The model under review builds one solid part; all positions refer to its coordinate system, in mm. A direction names the side the tool comes from. Give positions to 0.01 mm unless a question says otherwise; leave off trailing zeros. Order: outer loops, then holes, each group sorted by start corner. A loop starts at its lowest first (then second) coordinate and runs counter-clockwise, first axis right, second up. Notation, with made-up numbers: (52.25, -37) - (93.25, -37) arc R16 ccw to (93.25, -6) - close; hole circle Ø10 at (59.25, 70.5). An arc over 180 degrees is marked (long way). Put each result on its own line as item: value.
```python
from build123d import *

# Parameters (mm, degrees)
SKETCH_1_R               = 9.5
EXTRUDE_1_DEPTH          = 108
SKETCH_2_R               = 6.35
EXTRUDE_2_DEPTH          = 11.5
SKETCH_3_R               = 11
EXTRUDE_3_DEPTH          = 8
SKETCH_4_R               = 9.5
EXTRUDE_4_DEPTH          = 1.6
SKETCH_5_R               = 11
EXTRUDE_5_DEPTH          = 14
SKETCH_6_R               = 9.5
EXTRUDE_6_DEPTH          = 4
SKETCH_7_R               = 14.25
EXTRUDE_7_DEPTH          = 16
CHAMFER_1_SIZE           = 1.5
CUT_EXTRUDE_1_DEPTH      = 195.148744523
CUT_EXTRUDE_1_DEPTH_BACK = 195.148744523
EXTRUDE_8_DEPTH          = 14
EXTRUDE_8_DEPTH_BACK     = 14
SKETCH_12_R              = 8
EXTRUDE_9_DEPTH          = 3.2
SKETCH_13_R              = 9.5
EXTRUDE_10_DEPTH         = 6.4
CHAMFER_2_SIZE           = 1.5
CHAMFER_2_SIZE2          = 2.598076211


with BuildPart() as part:
    # Sketch 1 → Extrude 1 (new body)
    with BuildSketch(Plane.XY):
        Circle(SKETCH_1_R)
    extrude(amount=EXTRUDE_1_DEPTH)

    # Sketch 2 → Extrude 2 (add)
    with BuildSketch(Plane.XY.offset(108)):
        Circle(SKETCH_2_R)
    extrude(amount=EXTRUDE_2_DEPTH)

    # Sketch 3 → Extrude 3 (add)
    with BuildSketch(Plane.XY.offset(119.5)):
        Circle(SKETCH_3_R)
    extrude(amount=EXTRUDE_3_DEPTH)

    # Sketch 4 → Extrude 4 (add)
    with BuildSketch(Plane.XY.offset(127.5)):
        Circle(SKETCH_4_R)
    extrude(amount=EXTRUDE_4_DEPTH)

    # Sketch 5 → Extrude 5 (add)
    with BuildSketch(Plane.XY.offset(129.1)):
        Circle(SKETCH_5_R)
    extrude(amount=EXTRUDE_5_DEPTH)

    # Sketch 6 → Extrude 6 (add)
    with BuildSketch(Plane.XY.offset(143.1)):
        Circle(SKETCH_6_R)
    extrude(amount=EXTRUDE_6_DEPTH)

    # Sketch 7 → Extrude 7 (add)
    with BuildSketch(Plane.XY.offset(147.1)):
        Circle(SKETCH_7_R)
    extrude(amount=EXTRUDE_7_DEPTH)

    # Chamfer 1
    chamfer_1_edges = [part.edges().sort_by_distance(p)[0] for p in [
        (-14.25, 0, 163.1),
    ]]
    chamfer(chamfer_1_edges, length=CHAMFER_1_SIZE)

    # Sketch 8 → Revolve 1 (revolve)
    with BuildSketch(Plane(origin=(0, 0, 0), x_dir=(0, 0, -1), z_dir=(1, 0, 0)), mode=Mode.PRIVATE) as revolve_1_sk:
        Polygon((-163.1, 6.35), (-164.7, 6.35), (-164.7, 9.5), (-166.3, 9.5), (-166.3, 6.35), (-167.9, 6.35), (-167.9, 9.5), (-169.5, 9.5), (-169.5, 6.35), (-171.1, 6.35), (-171.1, 9.5), (-172.7, 9.5), (-172.7, 6.35), (-193.1, 6.35), (-193.1, 0), (-163.1, 0), align=None)
    revolve(revolve_1_sk.sketch.rotate(Axis((0, 0, 193.1), (0, 0, -1)), 90), axis=Axis((0, 0, 193.1), (0, 0, -1)))

    # Sketch 9 → Cut-Extrude 1 (cut, two sides: drawn at the far end of the back side and taken through both)
    with BuildSketch(Plane(origin=(0, 0, 0), x_dir=(0, 0, -1), z_dir=(1, 0, 0)).offset(-CUT_EXTRUDE_1_DEPTH_BACK)):
        Polygon((-179.653682132, -6.35), (-188.546317868, 6.35), (-193.1, 6.35), (-193.1, -6.35), align=None)
    extrude(amount=CUT_EXTRUDE_1_DEPTH + CUT_EXTRUDE_1_DEPTH_BACK, mode=Mode.SUBTRACT)

    # Sketch 10 → Extrude 8 (add, two sides: drawn at the far end of the back side and taken through both)
    with BuildSketch(Plane(origin=(0, 0, 0), x_dir=(0, 0, -1), z_dir=(1, 0, 0)).offset(-EXTRUDE_8_DEPTH_BACK)):
        Polygon((-176.815579258, -10.403230962), (-191.384420742, 10.403230962), (-215.688134824, -6.614412844), (-201.119293341, -27.420874769), align=None)
    extrude(amount=EXTRUDE_8_DEPTH + EXTRUDE_8_DEPTH_BACK)

    # Sketch 12 → Extrude 9 (add)
    with BuildSketch(Plane(origin=(0, 76.095474781, 53.282625065), x_dir=(1, 0, 0), z_dir=(0, -0.8191520442889946, -0.5735764363510424))):
        with Locations(Location((0, 165.640569636, 0), (0, 0, 270))):
            Circle(SKETCH_12_R)
    extrude(amount=EXTRUDE_9_DEPTH)

    # Sketch 13 → Extrude 10 (add)
    with BuildSketch(Plane(origin=(0, 73.474188239, 51.447180469), x_dir=(1, 0, 0), z_dir=(0, -0.8191520442889944, -0.5735764363510425))):
        with Locations(Location((0, 165.640569636, 0), (0, 0, 270))):
            Circle(SKETCH_13_R)
    extrude(amount=EXTRUDE_10_DEPTH)

    # Chamfer 2
    chamfer_2_edges = [part.edges().sort_by_distance(p)[0] for p in [
        (-14.25, 0, 147.1),
    ]]
    chamfer_2_side = [part.faces().sort_by_distance(p)[0] for p in [
        (-13.846949135, 0, 147.1),
    ]]
    chamfer(chamfer_2_edges, length=CHAMFER_2_SIZE, length2=CHAMFER_2_SIZE2, reference=chamfer_2_side[0])


solid = part.part
```
(1) Take a section at B-B, the plane z = 157. Write out the cut boundary in (x, y), then the cut area to 3 significant figures.
The answers:
outline: circle Ø28.5 at (0, 0)
area: 638 mm^2
(2) Wall thickness on L1, parallel to Z at x = -6, y = -6; L2, parallel to Z at x = -5, y = 9; L3, parallel to Y at x = 5, z = 177: over which ranges is each line inside the solid? List them lowest first.
The answers:
L1: 0 to 108, 119.5 to 163.1, 164.7 to 166.3, 167.9 to 169.5, 171.1 to 172.7, 179.9 to 214.81
L2: 119.5 to 127.5, 129.1 to 143.1, 147.1 to 163.1, 190.4 to 193.39
L3: -22.25 to -21.92, -10.53 to -10.14, -3.91 to 3.91
(3) For faces 1 (the cylindrical face through (-2.38, -10.74, 136)), 2 (the cylindrical face through (-5.04, 3.86, 170.31)), list the 3-axis set-ups (+Z, -Z, +X, -X, +Y, -Y) from which the entire face can be reached by the end or side of a thin tool; tool diameter is ignored.
The answers:
face 1: -Z
face 2: none
(4) Clearance check with flat-ended pins moving along their axes: pin 1 Ø4 at (y, z) = (-7.5, 85) entering from +X; pin 2 Ø2 at (x, z) = (1.5, 81) entering from +Y; pin 3 Ø2 at (x, y) = (-3, -16) entering from +Z; pin 4 Ø10 at (y, z) = (-27.5, 171) entering from -X. State where each tip first meets the part, or that it passes through.
The answers:
pin 1: x = 7.75
pin 2: y = 9.49
pin 3: z = 209.82
pin 4: through
(5) The part is to be moulded in two halves that separate along Z. For faces 3 (the flat face through (14, -8, 197)), 4 (the flat face through (2, 6.2, 166.3)), 5 (the flat face through (0, 0, 0)), say which applies: pulls with the +Z half, pulls with the -Z half, needs draft (parallel to the pull), parting line crosses it, or undercut.
The answers:
face 3: needs draft
face 4: undercut
face 5: pulls with the -Z half
(6) Take a section at A-A, the plane z = 22.5. Write out the cut boundary in (x, y).
The answers:
outline: circle Ø19 at (0, 0)
